from build123d import *

# Parameters (mm, degrees)
SKETCH1_R           = 4
BOSS_EXTRUDE1_DEPTH = 8
BOSS_EXTRUDE2_START = -8
SKETCH2_R           = 4
BOSS_EXTRUDE2_DEPTH = 8
FILLET1_R           = 5
SKETCH3_R           = 1.5
CUT_EXTRUDE1_DEPTH  = 19
SKETCH4_R           = 1.5
SKETCH4_R_2         = 12
CUT_EXTRUDE2_DEPTH  = 19
FILLET2_R           = 100


with BuildPart() as part:
    # Sketch1 → Boss-Extrude1 (new body)
    with BuildSketch(Plane(origin=(0, 0, 0), x_dir=(1, 0, 0), z_dir=(0, 1, 0))):
        with BuildLine():
            Line((0, -17.5), (126.259093916, -17.5))
            ThreePointArc((126.259093916, -17.5), (162.25, 0), (126.259093916, 17.5))
            Line((126.259093916, 17.5), (0, 17.5))
            ThreePointArc((0, 17.5), (-17.5, 0), (0, -17.5))
        make_face()
        with Locations(Location((140, 0, 0), (0, 0, 270))):
            Circle(SKETCH1_R, mode=Mode.SUBTRACT)
        with Locations(Location((0, 0, 0), (0, 0, 270))):
            Circle(SKETCH1_R, mode=Mode.SUBTRACT)
    extrude(amount=BOSS_EXTRUDE1_DEPTH)

    # Sketch2 → Boss-Extrude2 (add)
    with BuildSketch(Plane(origin=(0, 8, 0), x_dir=(1, 0, 0), z_dir=(0, 1, 0)).offset(BOSS_EXTRUDE2_START)):
        with BuildLine():
            Line((0, 22.5), (-77.5, 22.5))
            Line((-77.5, 22.5), (-77.5, -22.5))
            Line((-77.5, -22.5), (0, -22.5))
            ThreePointArc((0, -22.5), (22.5, 0), (0, 22.5))
        make_face()
        with BuildLine():
            ThreePointArc((-65, -14), (-63.5, -15.5), (-65, -17))
            Line((-65, -17), (-70, -17))
            ThreePointArc((-70, -17), (-71.5, -15.5), (-70, -14))
            Line((-70, -14), (-65, -14))
        make_face(mode=Mode.SUBTRACT)
        with BuildLine():
            Line((-39, -14), (-38, -14))
            Line((-38, -14), (-34, -14))
            ThreePointArc((-34, -14), (-32.5, -15.5), (-34, -17))
            Line((-34, -17), (-39, -17))
            ThreePointArc((-39, -17), (-40.5, -15.5), (-39, -14))
        make_face(mode=Mode.SUBTRACT)
        with BuildLine():
            ThreePointArc((-65, 17), (-63.5, 15.5), (-65, 14))
            Line((-65, 14), (-70, 14))
            ThreePointArc((-70, 14), (-71.5, 15.5), (-70, 17))
            Line((-70, 17), (-65, 17))
        make_face(mode=Mode.SUBTRACT)
        with BuildLine():
            ThreePointArc((-34, 17), (-32.5, 15.5), (-34, 14))
            Line((-34, 14), (-39, 14))
            ThreePointArc((-39, 14), (-40.5, 15.5), (-39, 17))
            Line((-39, 17), (-34, 17))
        make_face(mode=Mode.SUBTRACT)
        with Locations(Location((0, 0, 0), (0, 0, 270))):
            Circle(SKETCH2_R, mode=Mode.SUBTRACT)
    extrude(amount=BOSS_EXTRUDE2_DEPTH)

    # Fillet1
    fillet1_edges = [part.edges().sort_by_distance(p)[0] for p in [
        (-77.5, 4, -22.5),
        (-77.5, 4, 22.5),
    ]]
    fillet(fillet1_edges, radius=FILLET1_R)

    # Sketch3 → Cut-Extrude1 (cut)
    with BuildSketch(Plane(origin=(0, 8, 0), x_dir=(1, 0, 0), z_dir=(0, 1, 0))):
        with Locations(Location((0, 12.5, 0), (0, 0, 270))):
            Circle(SKETCH3_R)
        with Locations(Location((12.5, 0, 0), (0, 0, 270))):
            Circle(SKETCH3_R)
        with Locations(Location((0, -12.5, 0), (0, 0, 270))):
            Circle(SKETCH3_R)
        with Locations(Location((-12.5, 0, 0), (0, 0, 270))):
            Circle(SKETCH3_R)
    extrude(amount=-CUT_EXTRUDE1_DEPTH, mode=Mode.SUBTRACT)

    # Sketch4 → Cut-Extrude2 (cut)
    with BuildSketch(Plane(origin=(0, 8, 0), x_dir=(1, 0, 0), z_dir=(0, 1, 0))):
        with Locations(Location((157.25, 0, 0), (0, 0, 270))):
            Circle(SKETCH4_R)
        with Locations(Location((140, -17.25, 0), (0, 0, 270))):
            Circle(SKETCH4_R)
        with Locations(Location((122.75, 0, 0), (0, 0, 270))):
            Circle(SKETCH4_R)
        with Locations(Location((140, 17.25, 0), (0, 0, 270))):
            Circle(SKETCH4_R)
        with Locations(Location((140, 0, 0), (0, 0, 270))):
            Circle(SKETCH4_R_2)
    extrude(amount=-CUT_EXTRUDE2_DEPTH, mode=Mode.SUBTRACT)

    # Fillet2
    fillet2_edges = [part.edges().sort_by_distance(p)[0] for p in [
        (126.259093916, 4, -17.5),
        (126.259093916, 4, 17.5),
        (14.142135624, 4, -17.5),
        (14.142135624, 4, 17.5),
    ]]
    fillet(fillet2_edges, radius=FILLET2_R)


solid = part.part
Build history of the part. All positions in model axes, mm. A direction names the side the tool comes from. Round coordinates to 2 decimals unless told otherwise and drop trailing zeros. Loops run counter-clockwise (first coordinate to the right, second up) from the corner with the lowest first, then second, coordinate; pieces in that order, holes last. Notation, with made-up numbers: (-13, -29) -> (43, -29) arc R20 cw to (43, -1) -> close; hole circle Ø11 at (-6.5, 37.5). An arc over 180 degrees is marked (long way). One line per item, written item: value. Start each with the question number.
Q1. Probe line 1 along X through (y, z) = (2.5, 2.5); line 2 along Z through (x, y) = (-33, 7.75); line 3 along Z through (x, y) = (157.25, 2.25). List the from-to ranges inside material, lowest first.
Q2. Cut at C-C on y = 4. Count the separate pieces of the cut face and the enclosed holes in it, plus the area to 3 significant figures.
Q3. Cut at B-B on x = 61. List the corners of the cut face in (y, z).
Q4. Drop flat-ended pins along their axis: pin 1 Ø2.5 at (x, y) = (75, 2.5) entering from -Z; pin 2 Ø2.5 at (x, y) = (79, 4.5) entering from +Z; pin 3 Ø1 at (x, y) = (123.5, 1.5) entering from +Z. Give the stop position or say it passes through.
Q5. Two-plate mould, pull along X, no slides. Class faces 1 (the face through (-37, 4, -17)), 2 (the face through (-76.07, 4.06, 21)), 3 (the face through (-37, 4, 22.5)): released by +X, released by -X, zero draft, split by the parting line, or undercut.
Q6. Cut at A-A on z = 8. List the corners of the cut face in (x, y), plus the area to 3 significant figures.
Q7. 3-axis set-ups, long thin cutter, end or side, ignore diameter. For faces 4 (the face through (3.259, 3.944, -22.263)), 5 (the face through (41, 8, 0)), 6 (the face through (-68, 4, 14)), 7 (the face through (20.554, 3.944, 18.497)): which of +Z, -Z, +X, -X, +Y, -Y reach the whole face in a straight line?
Computed:
1. line 1: -77.5 to -3.12, 3.12 to 128.26, 151.74 to 162.11
1. line 2: -22.5 to -16.62, -14.38 to 14.38, 16.62 to 22.5
1. line 3: -14.05 to -1.5, 1.5 to 14.05
2. separate pieces: 1
2. enclosed holes: 14
2. area: 8,770 mm²
3. outline: (0, -17.5) -> (8, -17.5) -> (8, 17.5) -> (0, 17.5) -> close
4. pin 1: z = -17.5
4. pin 2: z = 17.5
4. pin 3: z = 19.09
5. face 1: undercut
5. face 2: released by -X
5. face 3: zero draft
6. outline: (-77.5, 0) -> (131.06, 0) -> (131.06, 8) -> (-77.5, 8) -> close; (148.94, 0) -> (160.76, 0) -> (160.76, 8) -> (148.94, 8) -> close
6. area: 1,760 mm²
7. face 4: -Z, +Y, -Y
7. face 5: +Z, -Z, +X, -X, +Y
7. face 6: +Y, -Y
7. face 7: +Z, +Y, -Y
